```python
from build123d import *

# Parameters (mm, degrees)
CYLINDER_R              = 10
CYLINDER_DEPTH          = 10
CYLINDER001_R           = 2
CYLINDER001_DEPTH       = 30
CYLINDER001_ROLL_ANGLE  = -90
CYLINDER002_R           = 11
CYLINDER002_DEPTH       = 7
CYLINDER002_PITCH_ANGLE = 90
CYLINDER003_R           = 10
CYLINDER003_DEPTH       = 10
CYLINDER003_PITCH_ANGLE = 90
BOX001_W                = 25
BOX001_H                = 10
BOX001_DEPTH            = 15
BOX002_W                = 10
BOX002_H                = 30
BOX002_DEPTH            = 40
BOX_W                   = 40
BOX_H                   = 30
BOX_DEPTH               = 10


with BuildPart() as cylinder:
    # Cylinder → Cylinder (new body)
    with BuildSketch(Plane.XY.offset(-5)):
        Circle(CYLINDER_R)
    extrude(amount=CYLINDER_DEPTH)


with BuildPart() as cylinder001:
    # Cylinder001 → Cylinder001 (new body)
    with BuildSketch(Plane.XY):
        Circle(CYLINDER001_R)
    extrude(amount=CYLINDER001_DEPTH)


with BuildPart() as cylinder001_1:
    # Cylinder001 roll: moved
    add(cylinder001.part.rotate(Axis((0, 0, 0), (1, 0, 0)), CYLINDER001_ROLL_ANGLE))


with BuildPart() as cylinder001_2:
    # Cylinder001 placement: moved
    add(cylinder001_1.part.moved(Location((-20, -15, 0))))


with BuildPart() as bearing_cylinder:
    # Cylinder002 → Cylinder002 (new body)
    with BuildSketch(Plane.XY):
        Circle(CYLINDER002_R)
    extrude(amount=CYLINDER002_DEPTH)


with BuildPart() as bearing_cylinder_1:
    # Cylinder002 pitch: moved
    add(bearing_cylinder.part.rotate(Axis((0, 0, 0), (0, 1, 0)), CYLINDER002_PITCH_ANGLE))


with BuildPart() as bearing_cylinder_2:
    # Cylinder002 placement: moved
    add(bearing_cylinder_1.part.moved(Location((-28.5, 0, 15))))


with BuildPart() as bearing_cylinder_outer:
    # Cylinder003 → Cylinder003 (new body)
    with BuildSketch(Plane.XY):
        Circle(CYLINDER003_R)
    extrude(amount=CYLINDER003_DEPTH)


with BuildPart() as bearing_cylinder_outer_1:
    # Cylinder003 pitch: moved
    add(bearing_cylinder_outer.part.rotate(Axis((0, 0, 0), (0, 1, 0)), CYLINDER003_PITCH_ANGLE))


with BuildPart() as bearing_cylinder_outer_2:
    # Cylinder003 placement: moved
    add(bearing_cylinder_outer_1.part.moved(Location((-30, 0, 15))))


with BuildPart() as negative_fusion:
    # Box001 → Box001 (new body)
    with BuildSketch(Plane(origin=(-30, -5, -5), x_dir=(1, 0, 0), z_dir=(0, 0, 1))):
        with Locations((12.5, 5)):
            Rectangle(BOX001_W, BOX001_H)
    extrude(amount=BOX001_DEPTH)

    # Fusion: union Cylinder, Cylinder001, Bearing Cylinder, Bearing Cylinder Outer
    add(cylinder.part)
    add(cylinder001_2.part)
    add(bearing_cylinder_2.part)
    add(bearing_cylinder_outer_2.part)


with BuildPart() as cube002:
    # Box002 → Box002 (new body)
    with BuildSketch(Plane(origin=(-30, -15, -5), x_dir=(1, 0, 0), z_dir=(0, 0, 1))):
        with Locations((5, 15)):
            Rectangle(BOX002_W, BOX002_H)
    extrude(amount=BOX002_DEPTH)


with BuildPart() as cut:
    # Box → Box (new body)
    with BuildSketch(Plane(origin=(-20, -15, -5), x_dir=(1, 0, 0), z_dir=(0, 0, 1))):
        with Locations((20, 15)):
            Rectangle(BOX_W, BOX_H)
    extrude(amount=BOX_DEPTH)

    # Fusion001: union Cube002
    add(cube002.part)

    # Cut: cut Negative Fusion
    add(negative_fusion.part, mode=Mode.SUBTRACT)


solid = cut.part
```
Part model, mm, in its own coordinate system. A direction names the side the tool comes from. Round coordinates to 2 decimals unless told otherwise and drop trailing zeros. Loops run counter-clockwise (first coordinate to the right, second up) from the corner with the lowest first, then second, coordinate; pieces in that order, holes last.
1. Flat gauge pins, fed straight in: pin 1 (12 mm diameter, centred on x = -9, y = -10.5, fed in from +Z); pin 2 (10.5 mm diameter, centred on y = 5, z = 11.5, fed in from +X). Where does each tip first touch, or does it go through?
Solutions:
pin 1: stops at z = 5
pin 2: stops at x = -20
2. Two-plate mould, pull along X, no slides. Class faces 1 (the face through (-28.5, 2, 25)), 2 (the face through (-30, -7, 24)), 3 (the face through (-21, 0, 25)): pulls with the +X half, pulls with the -X half, needs draft (parallel to the pull), parting line crosses it, or undercut.
Solutions:
face 1: undercut
face 2: pulls with the -X half
face 3: needs draft
3. 3-axis set-ups, long thin cutter, end or side, ignore diameter. For faces 4 (the face through (-11, 7, -5)), 5 (the face through (9, 7, 5)), 6 (the face through (-17, -5, 1)), 7 (the face through (-25, 0, 26)), 8 (the face through (-16, 15, 1)): which of +Z, -Z, +X, -X, +Y, -Y reach the whole face in a straight line?
Solutions:
face 4: -Z, +X, -X, +Y, -Y
face 5: +Z, +X, +Y, -Y
face 6: -Z, -X
face 7: none
face 8: +Z, -Z, +X, -X, +Y
4. Slice it at B-B (y = 0). Give the cut face in (x, z), and give its area (3 significant figures).
Solutions:
outline: (-30, 25) - (-28.5, 25) - (-28.5, 26) - (-21.5, 26) - (-21.5, 25) - (-20, 25) - (-20, 35) - (-30, 35) - close; (10, -5) - (20, -5) - (20, 5) - (10, 5) - close
area: 193 mm2
5. Slice it at C-C (y = -11.75). Give the cut face in (x, z), and give its area (3 significant figures).
Solutions:
outline: (-30, -5) - (20, -5) - (20, 5) - (-20, 5) - (-20, 35) - (-30, 35) - close; hole circle Ø4 at (-20, 0)
area: 787 mm2
6. Drill centre lines: line 1 along Y through (x, z) = (-26, 15); line 2 along Y through (x, z) = (0, 2.25); line 3 along X through (y, z) = (-7, 7). Where is each one in solid material? Low to high.
Solutions:
line 1: y = -15 to -11, 11 to 15
line 2: y = -15 to -10, 10 to 15
line 3: x = -30 to -28.5, -21.5 to -20
7. Slice it at D-D (x = 0). Give the cut face in (y, z), and give its area (3 significant figures).
Solutions:
outline: (-15, -5) - (-10, -5) - (-10, 5) - (-15, 5) - close; (10, -5) - (15, -5) - (15, 5) - (10, 5) - close
area: 100 mm2
8. Slice it at A-A (z = 15). Give the cut face in (x, y), and give its area (3 significant figures).
Solutions:
outline: (-30, -15) - (-20, -15) - (-20, -10) - (-21.5, -10) - (-21.5, -11) - (-28.5, -11) - (-28.5, -10) - (-30, -10) - close; (-30, 10) - (-28.5, 10) - (-28.5, 11) - (-21.5, 11) - (-21.5, 10) - (-20, 10) - (-20, 15) - (-30, 15) - close
area: 86.0 mm2
